CAD build for the part. Positions are in the model's coordinates, mm. Face numbers are marked on the shaded views. A direction names the side the tool comes from. Give positions to 0.01 mm unless a question says otherwise; leave off trailing zeros. Write each loop counter-clockwise with the first axis right and the second up, starting at its lowest first coordinate (ties: lowest second). Pieces come first, ordered by that corner, then holes. Notation, with made-up numbers: (82, 23.5) - (111, 23.5) arc R25 cw to (111, 52.5) - close; hole circle Ø1 at (-1.75, -8). An arc over 180 degrees is marked (long way). Put each result on its own line as item: value. Start each with the question number.
1. Drop flat-ended pins along their axis: pin 1 (5 mm diameter, centred on y = -4.5, z = 43, fed in from +X); pin 2 (17 mm diameter, centred on x = -17, y = 3.5, fed in from -Z); pin 3 (5 mm diameter, centred on x = 7.5, y = -9.5, fed in from -Z); pin 4 (10 mm diameter, centred on x = -5.5, z = -23, fed in from -Y). Give the stop position or say it passes through.
2. Cut at B-B on z = -34. List the corners of the cut face in (x, y), and give its area (3 significant figures).
3. Cut at C-C on y = 0. List the corners of the cut face in (x, z).
4. Tool access for the marked faces 1 and 2: list every direction of +Z, -Z, +X, -X, +Y, -Y with a clear straight run to the whole face (end or side of a thin tool).
5. Cut at D-D on z = 18. List the corners of the cut face in (x, y), and give its area (3 significant figures).
6. Cut at A-A on x = -12.7. List the corners of the cut face in (y, z).
7. Wall check: line 1 (Y direction, x = -12, z = -32); line 2 (Y direction, x = -12.7, z = -49); line 3 (X direction, y = -4, z = -23). Give the ranges that are in metal, low to high.
8. Mould opens along X. For the marked faces 3 and 4 say: +X half, -X half, draft (parallel to the pull), parting line (faces both ways), or undercut.
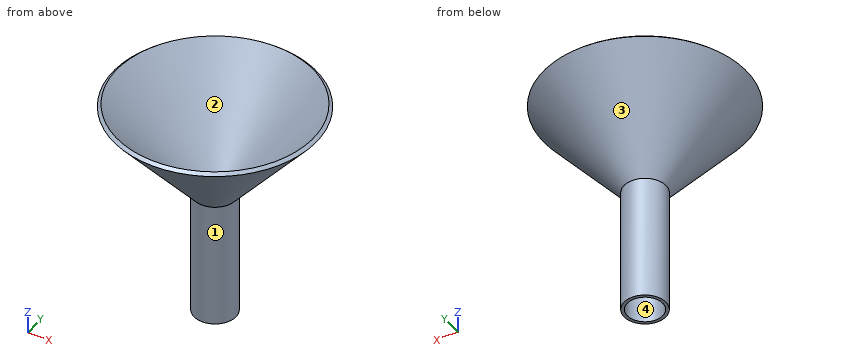
from build123d import *

# Parameters (mm, degrees)
F2_R     = 10.7682779898
F3_DEPTH = 25.4
F4_DEPTH = 25.4
F5_DEPTH = 25.4


with BuildPart() as f1:
    # F0 (on Front) → F1 (revolve)
    with BuildSketch(Plane.XZ):
        Polygon((0, -75.7813751698), (0, 0), (48.6775934706, 56.0841891061), (46.7580937851, 57.7373997368), (-2.9694908299, 0), (-12.7, 0), (-12.7, -75.7813751698), align=None)
    revolve(axis=Axis((-12.7, 0, -37.8906875849), (0, 0, 1)))

    # F2 (on face) → F3 (cut)
    with BuildSketch(Plane(origin=(0, 0, -75.7813751698), x_dir=(1, 0, 0), z_dir=(0, 0, -1))):
        with Locations((-12.7, 0)):
            Circle(F2_R)
    extrude(amount=-F3_DEPTH, mode=Mode.SUBTRACT)

    # F4 (cut): a face of the model
    f4_faces = [f1.faces().sort_by_distance(p)[0] for p in [
        (-12.7, 0, -50.3813751698),
    ]]
    extrude(f4_faces, amount=-F4_DEPTH, mode=Mode.SUBTRACT)

    # F5 (cut): a face of the model
    f5_faces = [f1.faces().sort_by_distance(p)[0] for p in [
        (-12.7, 0, -24.9813751698),
    ]]
    extrude(f5_faces, amount=-F5_DEPTH, mode=Mode.SUBTRACT)


solid = f1.part
Report:
1. pin 1: stops at x = 39.31
1. pin 2: stops at z = -75.78
1. pin 3: stops at z = 8.21
1. pin 4: stops at y = -12.51
2. outline: circle Ø25.4 at (-12.7, 0); hole circle Ø21.54 at (-12.7, 0)
2. area: 142 mm²
3. outline: (-74.08, 56.08) - (-25.4, 0) - (-25.4, -75.78) - (-23.47, -75.78) - (-23.47, 0.42) - (-22.79, 0.42) - (-72.16, 57.74) - close; (-2.61, 0.42) - (-1.93, 0.42) - (-1.93, -75.78) - (0, -75.78) - (0, 0) - (48.68, 56.08) - (46.76, 57.74) - close
4. face 1: -Z
4. face 2: +Z
5. outline: circle Ø56.65 at (-12.7, 0); hole circle Ø50.47 at (-12.7, 0)
5. area: 520 mm²
6. outline: (-61.38, 56.08) - (-12.7, 0) - (-12.7, -75.78) - (-10.77, -75.78) - (-10.77, 0.42) - (-10.09, 0.42) - (-59.46, 57.74) - close; (10.09, 0.42) - (10.77, 0.42) - (10.77, -75.78) - (12.7, -75.78) - (12.7, 0) - (61.38, 56.08) - (59.46, 57.74) - close
7. line 1: y = -12.68 to -10.75, 10.75 to 12.68
7. line 2: y = -12.7 to -10.77, 10.77 to 12.7
7. line 3: x = -24.75 to -22.7, -2.7 to -0.65
8. face 3: parting line
8. face 4: undercut
